The figure shows three views and two pictorial views of one solid part (mm, origin at its lowest corner). Answer the questions. A direction names the side the tool comes from. Give positions to 0.01 mm unless a question says otherwise; leave off trailing zeros. Loops run counter-clockwise (first coordinate to the right, second up) from the corner with the lowest first, then second, coordinate; pieces in that order, holes last. Notation, with made-up numbers: M 20,39.25 L 40,39.25 A16 ccw 40,62.25 Z; hole C 38,81.5 d8. An arc over 180 degrees is marked long. One line per item, written item: value. Start each with the question number.
Q1. A cutting plane is placed at C-C, the plane x = 14.5. Determine the outline of the cut face in (y, z).
Q2. Flat-ended cylindrical pins translate along their axes: pin 1 (3 mm diameter, centred on x = 2.5, z = 1.5, fed in from -Y); pin 2 (3 mm diameter, centred on x = 26.25, y = 14.5, fed in from +Z); pin 3 (2 mm diameter, centred on x = 21.5, y = 14.5, fed in from +Z); pin 4 (3.5 mm diameter, centred on y = 2.5, z = 3, fed in from -X). Find the tip coordinate at first contact, or state that the pin passes through.
Q3. A cutting plane is placed at D-D, the plane z = 4.5. Determine the outline of the cut face in (x, y).
Q4. A cutting plane is placed at B-B, the plane y = 14.5. Determine the outline of the cut face in (x, z), and give its area (3 significant figures).
Q5. For the marked faces 1, 2 and 3, determine the directions among +Z, -Z, +X, -X, +Y, -Y from which every point of the face is accessible in a straight line to the end or side of a thin tool.
Q6. Consider L1, parallel to X at y = 2.25, z = 5.5; L2, parallel to Y at x = 8.75, z = 1.9; L3, parallel to Z at x = 4.5, y = 14.25. Determine where each line is inside the solid, lowest interval first.
Q7. A cutting plane is placed at A-A, the plane x = 8.75. Determine the outline of the cut face in (y, z), and give its area (3 significant figures).
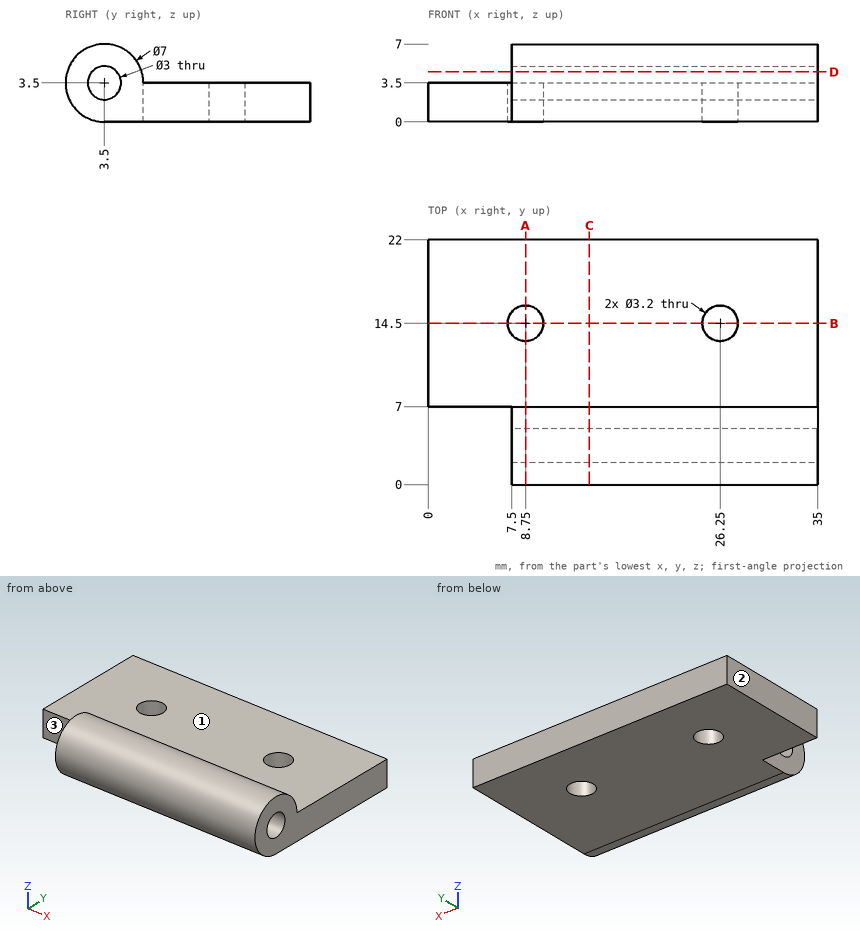
Answer block:
1. outline: M 3.5,0 L 22,0 L 22,3.5 L 7,3.5 A3.5 ccw long Z; hole C 3.5,3.5 d3
2. pin 1: y = 7
2. pin 2: through
2. pin 3: z = 3.5
2. pin 4: x = 7.5
3. outline: M 7.5,0.15 L 35,0.15 L 35,2.38 L 7.5,2.38 Z; M 7.5,4.62 L 35,4.62 L 35,6.85 L 7.5,6.85 Z
4. outline: M 0,0 L 7.15,0 L 7.15,3.5 L 0,3.5 Z; M 10.35,0 L 24.65,0 L 24.65,3.5 L 10.35,3.5 Z; M 27.85,0 L 35,0 L 35,3.5 L 27.85,3.5 Z
4. area: 100 mm^2
5. face 1: +Z, +X, -X, +Y
5. face 2: +Z, -Z, -X, +Y, -Y
5. face 3: +Z, -Z, -X, -Y
6. L1: 7.5 to 35
6. L2: 0.39 to 12.9, 16.1 to 22
6. L3: 0 to 3.5
7. outline: M 3.5,0 L 12.9,0 L 12.9,3.5 L 7,3.5 A3.5 ccw long Z; M 16.1,0 L 22,0 L 22,3.5 L 16.1,3.5 Z; hole C 3.5,3.5 d3
7. area: 75.3 mm^2
